```python
from build123d import *

# Parameters (mm, degrees)
PAD003_DEPTH                = 100
PAD002_DEPTH                = 100
PAD001_DEPTH                = 100
CYLINDER009_R               = 13
CYLINDER009_DEPTH           = 400
CYLINDER009_ROLL_ANGLE      = -23.419924
CYLINDER009_PITCH_ANGLE     = -34.667447
CYLINDER009_PLACEMENT_ANGLE = 7.402808
CYLINDER012_R               = 13
CYLINDER012_DEPTH           = 400
CYLINDER012_PLACEMENT_ANGLE = 41
CYLINDER013_R               = 13
CYLINDER013_DEPTH           = 400
CYLINDER013_ROLL_ANGLE      = -23.419924
CYLINDER013_PITCH_ANGLE     = 34.667447
CYLINDER013_PLACEMENT_ANGLE = -7.402808


with BuildPart() as body004:
    # Sketch005 → Pad003 (new body)
    with BuildSketch(Plane.XY):
        with BuildLine():
            ThreePointArc((86.165943, -28.96332), (78.724727, 45.451743), (18, 89.103555))
            Line((18, 14.317821), (18, 89.103555))
            ThreePointArc((21.399597, 8.429547), (19.918584, 11.5), (18, 14.317821))
            Line((21.399597, 8.429547), (86.165943, -28.96332))
        make_face()
    extrude(amount=PAD003_DEPTH)


with BuildPart() as body003:
    # Sketch006 → Pad002 (new body)
    with BuildSketch(Plane.XY):
        with BuildLine():
            Line((-3.399597, -22.747368), (-68.165943, -60.140235))
            ThreePointArc((-68.165943, -60.140235), (0, -90.903485), (68.165943, -60.140235))
            Line((3.399597, -22.747368), (68.165943, -60.140235))
            ThreePointArc((-3.399597, -22.747368), (0, -23), (3.399597, -22.747368))
        make_face()
    extrude(amount=PAD002_DEPTH)


with BuildPart() as fusion002:
    # Sketch004 → Pad001 (new body)
    with BuildSketch(Plane.XY):
        with BuildLine():
            Line((-21.399597, 8.429547), (-86.165943, -28.96332))
            ThreePointArc((-18, 89.103555), (-78.724727, 45.451743), (-86.165943, -28.96332))
            Line((-18, 14.317821), (-18, 89.103555))
            ThreePointArc((-18, 14.317821), (-19.918584, 11.5), (-21.399597, 8.429547))
        make_face()
    extrude(amount=PAD001_DEPTH)

    # Fusion002: union Body004, Body003
    add(body004.part)
    add(body003.part)


with BuildPart() as fusion002_1:
    # Fusion002 placement: moved
    add(fusion002.part.moved(Location((0, 0, 240))))


with BuildPart() as cylinder009:
    # Cylinder009 → Cylinder009 (new body)
    with BuildSketch(Plane.XY):
        Circle(CYLINDER009_R)
    extrude(amount=CYLINDER009_DEPTH)


with BuildPart() as cylinder009_1:
    # Cylinder009 roll: moved
    add(cylinder009.part.rotate(Axis((0, 0, 0), (1, 0, 0)), CYLINDER009_ROLL_ANGLE))


with BuildPart() as cylinder009_2:
    # Cylinder009 pitch: moved
    add(cylinder009_1.part.rotate(Axis((0, 0, 0), (0, 1, 0)), CYLINDER009_PITCH_ANGLE))


with BuildPart() as cylinder009_3:
    # Cylinder009 placement: moved
    add(cylinder009_2.part.moved(Location((250, -144.34, 0))).rotate(Axis((250, -144.34, 0), (0, 0, 1)), CYLINDER009_PLACEMENT_ANGLE))


with BuildPart() as cylinder012:
    # Cylinder012 → Cylinder012 (new body)
    with BuildSketch(Plane.XY):
        Circle(CYLINDER012_R)
    extrude(amount=CYLINDER012_DEPTH)


with BuildPart() as cylinder012_1:
    # Cylinder012 placement: moved
    add(cylinder012.part.moved(Location((0, 288.68, 0))).rotate(Axis((0, 288.68, 0), (1, 0, 0)), CYLINDER012_PLACEMENT_ANGLE))


with BuildPart() as tripod001:
    # Cylinder013 → Cylinder013 (new body)
    with BuildSketch(Plane.XY):
        Circle(CYLINDER013_R)
    extrude(amount=CYLINDER013_DEPTH)


with BuildPart() as tripod001_1:
    # Cylinder013 roll: moved
    add(tripod001.part.rotate(Axis((0, 0, 0), (1, 0, 0)), CYLINDER013_ROLL_ANGLE))


with BuildPart() as tripod001_2:
    # Cylinder013 pitch: moved
    add(tripod001_1.part.rotate(Axis((0, 0, 0), (0, 1, 0)), CYLINDER013_PITCH_ANGLE))


with BuildPart() as tripod001_3:
    # Cylinder013 placement: moved
    add(tripod001_2.part.moved(Location((-250, -144.34, 0))).rotate(Axis((-250, -144.34, 0), (0, 0, 1)), CYLINDER013_PLACEMENT_ANGLE))

    # Fusion001: union Cylinder009, Cylinder012
    add(cylinder009_3.part)
    add(cylinder012_1.part)


with BuildPart() as f_41_tripodsupport:
    # Sketch001 → Revolution002 (revolve)
    with BuildSketch(Plane.XZ):
        with BuildLine():
            Line((-49.269007, 313), (-13.5, 313))
            ThreePointArc((-13, 312.5), (-13.146447, 312.853553), (-13.5, 313))
            Line((-13, 312.5), (-13, 262.929281))
            Line((-13, 262.929281), (-87, 262.929281))
            Line((-87, 262.929281), (-49.269007, 313))
        make_face()
    revolve(axis=Axis((0, 0, 0), (0, 0, 1)))

    # Cut004: cut Tripod001
    add(tripod001_3.part, mode=Mode.SUBTRACT)

    # Cut005: cut Fusion002
    add(fusion002_1.part, mode=Mode.SUBTRACT)


solid = f_41_tripodsupport.part
```
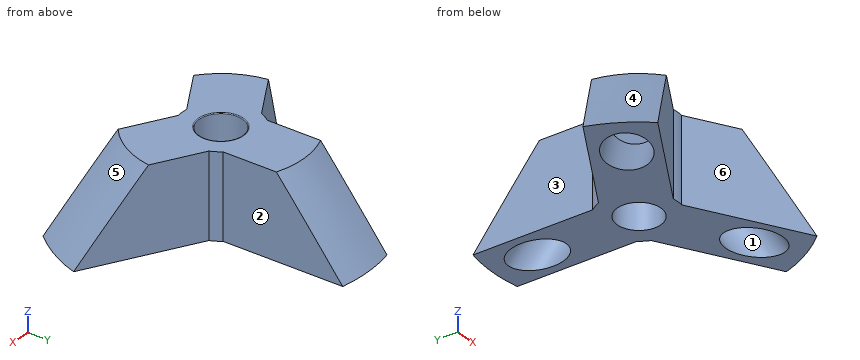
CAD build for the part. Positions are in the model's coordinates, mm. Face numbers are marked on the shaded views. A direction names the side the tool comes from. Give positions to 0.01 mm unless a question says otherwise; leave off trailing zeros. Write each loop counter-clockwise with the first axis right and the second up, starting at its lowest first coordinate (ties: lowest second). Pieces come first, ordered by that corner, then holes. Notation, with made-up numbers: M 70,41.25 L 79,41.25 A18 ccw 79,69.25 Z; hole C 29.25,86.25 d6. An arc over 180 degrees is marked long. Return JSON: item names as keys, results as strings. Group by question number.
(1) Band-saw the part on B-B (y = -5.5). State how many separate pieces and enclosed holes the cut face has, and give its area (3 significant figures).
(2) Mould opens along X. For the marked faces 4, 5 and 6 say: pulls with the +X half, pulls with the -X half, needs draft (parallel to the pull), parting line crosses it, or undercut.
(3) Drill centre lines: L1, parallel to Y at x = 23, z = 281.5; L2, parallel to X at y = 0, z = 286.5; L3, parallel to Y at x = -18.5, z = 290. Where is each one in solid material? Low to high. Write a range as [from, to].
(4) Flat gauge pins, fed straight in: pin 1 Ø5 at (y, z) = (40.5, 294) entering from +X; pin 2 Ø8 at (x, z) = (41.5, 297.5) entering from -Y; pin 3 Ø12 at (x, z) = (53.5, 294) entering from +Y; pin 4 Ø15.5 at (x, y) = (0, 0) entering from +Z. Where does each tip first touch, or does it go through?
(5) Band-saw the part on A-A (x = 0). Give the cut face in (y, z).
(6) 3-axis set-ups, long thin cutter, end or side, ignore diameter. For the marked faces 1, 2 and 3: which of +Z, -Z, +X, -X, +Y, -Y reach the whole face in a straight line?
Entries:
{
 "1": {"separate pieces": "2", "enclosed holes": "2", "area": "3,010 mm^2"},
 "2": {"face 4": "pulls with the -X half", "face 5": "pulls with the +X half", "face 6": "undercut"},
 "3": {"L1": "y = [-34.06, -24.98], [-13.66, 7.51]", "L2": "x = [-36, -13], [13, 36]", "L3": "y = [-31.47, -24.39], [-7.68, 13.67]"},
 "4": {"pin 1": "stops at x = 18", "pin 2": "stops at y = -46.02", "pin 3": "stops at y = -6.64", "pin 4": "passes through"},
 "5": {"outline": "M -23,262.93 L -13,262.93 L -13,312.5 A0.5 ccw -13.5,313 L -23,313 Z; M 13,262.93 L 42.89,262.93 L 16.45,293.36 L 36.07,310.41 L 77.34,262.93 L 87,262.93 L 49.27,313 L 13.5,313 A0.5 ccw 13,312.5 Z"},
 "6": {"face 1": "none", "face 2": "+Z, -Z, +X, +Y", "face 3": "+Z, -Z, -X, +Y"}
}
